Design review of the part built by this model. Coordinates are the model's own, in mm. Coordinates: 2 decimals unless noted, no trailing zeros. Order: outer loops, then holes, each group sorted by start corner. A loop starts at its lowest first (then second) coordinate and runs counter-clockwise, first axis right, second up. Notation, with made-up numbers: (-13, -7.75) - (9, -7.75) arc R27 cw to (9, 8.25) - close; hole circle Ø11 at (-19.5, -36.75). An arc over 180 degrees is marked (long way). Write item = value, one per line. Start each with the question number.
```python
from build123d import *

# Parameters (mm, degrees)
SKETCH1_R           = 6
SKETCH1_R_2         = 3
BOSS_EXTRUDE1_DEPTH = 9
BOSS_EXTRUDE2_START = -3
SKETCH2_R           = 10
SKETCH2_R_2         = 3
BOSS_EXTRUDE2_DEPTH = 3
CHAMFER1_SIZE       = 2
FILLET1_R           = 2


with BuildPart() as part:
    # Sketch1 → Boss-Extrude1 (new body)
    with BuildSketch(Plane(origin=(0, 0, 0), x_dir=(1, 0, 0), z_dir=(0, 1, 0))):
        with Locations(Location((0, 0, 0), (0, 0, 270))):
            Circle(SKETCH1_R)
        with Locations(Location((0, 0, 0), (0, 0, 270))):
            Circle(SKETCH1_R_2, mode=Mode.SUBTRACT)
    extrude(amount=BOSS_EXTRUDE1_DEPTH)

    # Sketch2 → Boss-Extrude2 (add)
    with BuildSketch(Plane(origin=(0, 9, 0), x_dir=(1, 0, 0), z_dir=(0, 1, 0)).offset(BOSS_EXTRUDE2_START)):
        with Locations(Location((0, 0, 0), (0, 0, 270))):
            Circle(SKETCH2_R)
        with Locations(Location((0, 0, 0), (0, 0, 270))):
            Circle(SKETCH2_R_2, mode=Mode.SUBTRACT)
    extrude(amount=BOSS_EXTRUDE2_DEPTH)

    # Chamfer1
    chamfer1_edges = [part.edges().sort_by_distance(p)[0] for p in [
        (0, 6, -6),
        (0, 6, -10),
    ]]
    chamfer(chamfer1_edges, length=CHAMFER1_SIZE - 0.0001)  # a hair under: the kernel refuses the full size

    # Fillet1
    fillet1_edges = [part.edges().sort_by_distance(p)[0] for p in [
        (0, 4.0001, -6),
    ]]
    fillet(fillet1_edges, radius=FILLET1_R)


solid = part.part
```
Item 1: Add section B-B on y = 7. Give the boundary of the cut face in (x, z), plus the area to 3 significant figures.
Item 2: Mouldability with a two-part tool opening along X and no side actions: class faces 1 (the cylindrical face through (1.802, 1.564, 5.723)), 2 (the flat face through (2.4, 9, 2.1)), 3 (the cylindrical face through (0.9, 4.44, 2.86)) as +X half, -X half, draft (parallel to the pull), parting line (faces both ways), or undercut.
Item 3: For P1, Ø4, axis at x = 2.5, y = 2.5, coming from the +Z side; P2, Ø10, axis at x = 3, z = -0.5, coming from the -Y side; P3, Ø2, axis at y = 5.5, z = -3, coming from the -X side; P4, Ø5.5, axis at x = 0, z = 0, coming from the +Y side, all flat-tipped, find the tip position at first contact; note any pin that passes through.
Item 4: For line 1 (X direction, y = 5.5, z = 0.25); line 2 (X direction, y = 2.5, z = 0); line 3 (Y direction, x = 5, z = 7.5), list the stretches that pass through material, from the lowest coordinate up.
Item 5: Add section A-A on y = 2.25. Give the boundary of the cut face in (x, z), plus the area to 3 significant figures.
Worked out:
q1.outline = circle Ø18 at (0, 0); hole circle Ø6 at (0, 0)
q1.area = 226 mm2
q2.face_1 = parting line
q2.face_2 = draft
q2.face_3 = undercut
q3.P1 = 6.14
q3.P2 = 0
q3.P3 = -8.01
q3.P4 = through
q4.line_1 = -7.5 to -2.99, 2.99 to 7.5
q4.line_2 = -6 to -3, 3 to 6
q4.line_3 = 7.01 to 9
q5.outline = circle Ø12 at (0, 0); hole circle Ø6 at (0, 0)
q5.area = 84.8 mm2
